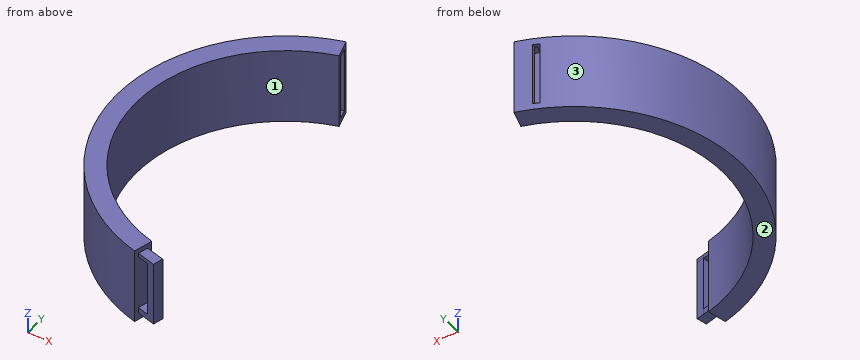
```python
from build123d import *

# Parameters (mm, degrees)
F1_DEPTH  = 20
F2_W      = 2.6613399386
F2_H      = 1.0413937271
F2_H_2    = 1.5042340383
F3_DEPTH  = 3
F5_DEPTH  = 2
F6_W      = 2.6971405605
F6_H      = 17.4564992776
F7_DEPTH  = 5
F9_W      = 1.6222847626
F9_H      = 16.6863657068
F10_DEPTH = 4.8


# Not quite as in the source:
# - ends of sketch curves that miss each other by under 0.0002 mm in the source are joined


with BuildPart() as f1:
    # F0 (on Top) → F1 (new body)
    with BuildSketch(Plane.XY):
        with BuildLine():
            ThreePointArc((0, -74.9042034149), (-28.4520233491, -37.4521017075), (0, 0))
            Line((0, 0), (-1.3406298741, 4.8169190701))
            ThreePointArc((-1.3406298741, 4.8169190701), (-33.4520231279, -37.4521017075), (-1.3406298741, -79.7211224851))
            Line((-1.3406298741, -79.7211224851), (0, -74.9042034149))
        make_face()
    extrude(amount=F1_DEPTH)

    # F2 (on face) → F3 (join)
    with BuildSketch(Plane(origin=(19.3483734862, -5.3849788907, 0), x_dir=(0.2681259867, 0.9633838567, 0), z_dir=(0.9633838567, -0.2681259867, 0))):
        with Locations((-74.7193582356, 18.2154309005)):
            Rectangle(F2_W, F2_H)
        with Locations((-74.7193582356, 2.5945375673)):
            Rectangle(F2_W, F2_H_2)
    extrude(amount=F3_DEPTH)

    # F4 (on face) → F5 (join)
    with BuildSketch(Plane(origin=(22.2385250561, -6.1893568507, 0), x_dir=(0.2681259867, 0.9633838567, 0), z_dir=(0.9633838567, -0.2681259867, 0))):
        Polygon((-73.3886882663, 17.6947340369), (-76.0500282049, 17.6947340369), (-76.0500282049, 1.8424974987), (-73.3886659145, 1.8424974987), align=None)
        Polygon((-73.3886659145, 18.736127764), (-76.0500282049, 18.736127764), (-76.0500282049, 17.6947340369), (-73.3886882663, 17.6947340369), align=None)
    extrude(amount=F5_DEPTH)

    # F6 (on face) → F7 (cut)
    with BuildSketch(Plane(origin=(0, 0, 0), x_dir=(-0.2681259867, 0.9633838567, 0), z_dir=(0.9633838567, 0.2681259867, 0))):
        with Locations((2.4999994203, 10.1498414879)):
            Rectangle(F6_W, F6_H)
    extrude(amount=-F7_DEPTH, mode=Mode.SUBTRACT)

    # F9 (on offset) → F10 (cut)
    with BuildSketch(Plane.XZ.offset(-4.7)):
        with Locations((-6.0561252758, 9.9340636516)):
            Rectangle(F9_W, F9_H)
    extrude(amount=F10_DEPTH, mode=Mode.SUBTRACT)


solid = f1.part
```
Can you work these out from the model? Positions are in its coordinate system, mm. Face numbers are marked on the shaded views. Coordinates: 2 decimals unless noted, no trailing zeros. Order: outer loops, then holes, each group sorted by start corner. A loop starts at its lowest first (then second) coordinate and runs counter-clockwise, first axis right, second up. Notation, with made-up numbers: (-2.5, 52.25) - (45.5, 52.25) arc R30 cw to (45.5, 89.25) - close; hole circle Ø6 at (42, -29). An arc over 180 degrees is marked (long way). Answer in a Markdown table with one row per item.
1. For pin 1 (1.7 mm diameter, centred on x = 0.5, y = -77.5, fed in from +Z); pin 2 (2 mm diameter, centred on y = -47, z = 9.5, fed in from +X); pin 3 (10 mm diameter, centred on x = -7, z = 14, fed in from +Y); pin 4 (2 mm diameter, centred on x = -3.5, y = 2, fed in from -Z), each with a flat end and sliding along its axis, tell me the tip position at first contact or that it passes through.
Reply:
| item | result |
|---|---|
| pin 1 | stops at z = 18.74 |
| pin 2 | stops at x = -26.99 |
| pin 3 | stops at y = 4.63 |
| pin 4 | stops at z = 0 |
2. Suppose I cut it at A-A (x = -9.5). Please give me the cut outline in (y, z), and give its area (3 significant figures).
Reply:
| item | result |
|---|---|
| outline | (-76.54, 0) - (-70.83, 0) - (-70.83, 20) - (-76.54, 20) - close; (-4.07, 0) - (1.64, 0) - (1.64, 20) - (-4.07, 20) - close |
| area | 228 mm^2 |
3. Suppose I cut it at C-C (x = -20). Please give me the cut outline in (y, z), and give its area (3 significant figures).
Reply:
| item | result |
|---|---|
| outline | (-69.07, 0) - (-61.65, 0) - (-61.65, 20) - (-69.07, 20) - close; (-13.25, 0) - (-5.84, 0) - (-5.84, 20) - (-13.25, 20) - close |
| area | 297 mm^2 |
4. If I drill on line 1 along Y through (x, z) = (-2, 13.5); line 2 along Y through (x, z) = (-21, 5); line 3 along Y through (x, z) = (-18.5, 6.75), over which ranges is the centre line in solid material (lowest first)?
Reply:
| item | result |
|---|---|
| line 1 | y = -79.53 to -74.29, -0.62 to 0.64, 3.44 to 4.63 |
| line 2 | y = -68.07 to -60.34, -14.56 to -6.83 |
| line 3 | y = -70.44 to -63.43, -11.48 to -4.46 |
5. Suppose I cut it at B-B (z = 6.75). Please give me the cut outline in (x, y).
Reply:
| item | result |
|---|---|
| outline | (-6.87, -0.1) - (-6.87, 2.87) arc R43.88 ccw to (-1.34, -79.72) - (0, -74.9) arc R38.88 cw to (0, 0) - (-0.31, 1.11) - (-5.13, -0.23) - (-5.24, 0.2) - (-5.24, -0.1) - close; (-5.24, 2.54) - (-1.03, 3.71) - (-1.34, 4.82) arc R43.88 ccw to (-5.24, 3.53) - close; (1.85, -79.45) - (3.77, -79.99) - (4.49, -77.43) - (2.56, -76.89) - close |
6. Suppose I cut it at D-D (y = -61.5). Please give me the cut outline in (x, z).
Reply:
| item | result |
|---|---|
| outline | (-26.27, 0) - (-20.12, 0) - (-20.12, 20) - (-26.27, 20) - close |
7. If we mould it in two halves opening along Y, with no side actions, what happens to the marked faces 1, 2 and 3? For each: pulls with the +Y half, pulls with the -Y half, needs draft (parallel to the pull), parting line crosses it, or undercut.
Reply:
| item | result |
|---|---|
| face 1 | undercut |
| face 2 | needs draft |
| face 3 | parting line crosses it |
